from build123d import *

# Parameters (mm, degrees)
F1_DEPTH = 1.25
F3_DEPTH = 4.75
F5_DEPTH = 2


with BuildPart() as f1:
    # F0 (on Top) → F1 (new body)
    with BuildSketch(Plane.XY):
        with BuildLine():
            ThreePointArc((5.9976509575, 42.832122093), (6.6456632834, 42.7363739632), (7.2921511628, 42.6308225515))
            Line((7.2921511628, 42.6308225515), (7.5029069767, 43.8629272495))
            ThreePointArc((7.5029069767, 43.8629272495), (6.7010150496, 43.9925720697), (5.8968902794, 44.1075581395))
            ThreePointArc((5.8968902794, 44.1075581395), (5.9741669577, 43.5561736795), (6, 43))
            ThreePointArc((6, 43), (5.9994127106, 42.9160528296), (5.9976509575, 42.832122093))
        make_face()
        with BuildLine():
            Line((-7.5029069767, 43.8629272495), (-7.2921511628, 42.6308225515))
            ThreePointArc((-7.2921511628, 42.6308225515), (-6.6456632834, 42.7363739632), (-5.9976509575, 42.832122093))
            ThreePointArc((-5.9976509575, 42.832122093), (-5.9813637313, 43.4725335051), (-5.8968902794, 44.1075581395))
            ThreePointArc((-5.8968902794, 44.1075581395), (-6.7010150496, 43.9925720697), (-7.5029069767, 43.8629272495))
        make_face()
        with BuildLine():
            ThreePointArc((1.2281761729, 43.2325581395), (3.6184570865, 43.0983673509), (5.9976509575, 42.832122093))
            ThreePointArc((5.9976509575, 42.832122093), (5.9994127106, 42.9160528296), (6, 43))
            ThreePointArc((6, 43), (5.9741669577, 43.5561736795), (5.8968902794, 44.1075581395))
            ThreePointArc((5.8968902794, 44.1075581395), (0, 44.5), (-5.8968902794, 44.1075581395))
            ThreePointArc((-5.8968902794, 44.1075581395), (-5.9813637313, 43.4725335051), (-5.9976509575, 42.832122093))
            ThreePointArc((-5.9976509575, 42.832122093), (-3.6184570865, 43.0983673509), (-1.2281761729, 43.2325581395))
            ThreePointArc((-1.2281761729, 43.2325581395), (0, 44.25), (1.2281761729, 43.2325581395))
        make_face()
        with BuildLine():
            ThreePointArc((5.1487358592, 39.9193313953), (5.9687994799, 39.804973719), (6.7863372093, 39.6737712763))
            Line((6.7863372093, 39.6737712763), (7.2921511628, 42.6308225515))
            ThreePointArc((7.2921511628, 42.6308225515), (6.6456632834, 42.7363739632), (5.9976509575, 42.832122093))
            ThreePointArc((5.9976509575, 42.832122093), (5.7603447969, 41.3211826125), (5.1487358592, 39.9193313953))
        make_face()
        with BuildLine():
            ThreePointArc((-5.1487358592, 39.9193313953), (0, 40.25), (5.1487358592, 39.9193313953))
            ThreePointArc((5.1487358592, 39.9193313953), (5.7603447969, 41.3211826125), (5.9976509575, 42.832122093))
            ThreePointArc((5.9976509575, 42.832122093), (3.6184570865, 43.0983673509), (1.2281761729, 43.2325581395))
            ThreePointArc((1.2281761729, 43.2325581395), (1.244532084, 43.1167899479), (1.25, 43))
            ThreePointArc((1.25, 43), (-0.1167899479, 41.755467916), (-1.2281761729, 43.2325581395))
            ThreePointArc((-1.2281761729, 43.2325581395), (-3.6184570865, 43.0983673509), (-5.9976509575, 42.832122093))
            ThreePointArc((-5.9976509575, 42.832122093), (-5.7603447969, 41.3211826125), (-5.1487358592, 39.9193313953))
        make_face()
        with BuildLine():
            Line((-7.2921511628, 42.6308225515), (-6.7863372093, 39.6737712763))
            ThreePointArc((-6.7863372093, 39.6737712763), (-5.9687994799, 39.804973719), (-5.1487358592, 39.9193313953))
            ThreePointArc((-5.1487358592, 39.9193313953), (-5.7603447969, 41.3211826125), (-5.9976509575, 42.832122093))
            ThreePointArc((-5.9976509575, 42.832122093), (-6.6456632834, 42.7363739632), (-7.2921511628, 42.6308225515))
        make_face()
        with BuildLine():
            Line((-6.7863372093, 39.6737712763), (-6.5755813953, 38.4416665782))
            ThreePointArc((-6.5755813953, 38.4416665782), (-5.4165900946, 38.6220215906), (-4.2526993305, 38.7674418605))
            ThreePointArc((-4.2526993305, 38.7674418605), (-4.7358693269, 39.3160426552), (-5.1487358592, 39.9193313953))
            ThreePointArc((-5.1487358592, 39.9193313953), (-5.9687994799, 39.804973719), (-6.7863372093, 39.6737712763))
        make_face()
        with BuildLine():
            ThreePointArc((-4.2526993305, 38.7674418605), (0, 39), (4.2526993305, 38.7674418605))
            ThreePointArc((4.2526993305, 38.7674418605), (4.7358693269, 39.3160426552), (5.1487358592, 39.9193313953))
            ThreePointArc((5.1487358592, 39.9193313953), (0, 40.25), (-5.1487358592, 39.9193313953))
            ThreePointArc((-5.1487358592, 39.9193313953), (-4.7358693269, 39.3160426552), (-4.2526993305, 38.7674418605))
        make_face()
        with BuildLine():
            ThreePointArc((4.2526993305, 38.7674418605), (5.4165900946, 38.6220215906), (6.5755813953, 38.4416665782))
            Line((6.5755813953, 38.4416665782), (6.7863372093, 39.6737712763))
            ThreePointArc((6.7863372093, 39.6737712763), (5.9687994799, 39.804973719), (5.1487358592, 39.9193313953))
            ThreePointArc((5.1487358592, 39.9193313953), (4.7358693269, 39.3160426552), (4.2526993305, 38.7674418605))
        make_face()
        with BuildLine():
            ThreePointArc((6.7863372093, 39.6737712763), (7.3721720875, 39.5690987857), (7.9563953488, 39.4557761684))
            Line((7.9563953488, 39.4557761684), (8.5494186047, 42.3965793611))
            ThreePointArc((8.5494186046, 42.3965793611), (7.9216507524, 42.5183483846), (7.2921511628, 42.6308225515))
            Line((7.2921511628, 42.6308225515), (6.7863372093, 39.6737712763))
        make_face()
        with BuildLine():
            Line((-8.5494186047, 42.3965793611), (-7.9563953488, 39.4557761684))
            ThreePointArc((-7.9563953488, 39.4557761684), (-7.3721720874, 39.5690987857), (-6.7863372093, 39.6737712763))
            Line((-6.7863372093, 39.6737712763), (-7.2921511628, 42.6308225515))
            ThreePointArc((-7.2921511628, 42.6308225515), (-7.9216507524, 42.5183483846), (-8.5494186046, 42.3965793611))
        make_face()
    extrude(amount=F1_DEPTH)

    # F2 (on Top) → F3 (join)
    with BuildSketch(Plane.XY):
        with BuildLine():
            ThreePointArc((6.0348837209, 42.8268920011), (7.2953245865, 42.6302796047), (8.5494186046, 42.3965793611))
            Line((8.5494186047, 42.3965793611), (8.7965116279, 43.6219140247))
            ThreePointArc((8.7965116279, 43.6219140247), (7.5061721179, 43.8623686106), (6.2093023256, 44.0646634462))
            Line((6.2093023256, 44.0646634462), (6.0348837209, 42.8268920011))
        make_face()
        with BuildLine():
            Line((-8.7965116279, 43.6219140247), (-8.5494186047, 42.3965793611))
            ThreePointArc((-8.5494186046, 42.3965793611), (-7.2953245865, 42.6302796047), (-6.0348837209, 42.8268920011))
            Line((-6.0348837209, 42.8268920011), (-6.2093023256, 44.0646634462))
            ThreePointArc((-6.2093023256, 44.0646634462), (-7.5061721179, 43.8623686106), (-8.7965116279, 43.6219140247))
        make_face()
    extrude(amount=F3_DEPTH)

    # F4 (on Top) → F5 (join)
    with BuildSketch(Plane.XY):
        with BuildLine():
            Line((-7.9563953488, 39.4557761684), (-7.7093023256, 38.2304415048))
            ThreePointArc((-7.7093023256, 38.2304415048), (-7.1432226437, 38.3402447862), (-6.5755813953, 38.4416665782))
            Line((-6.5755813953, 38.4416665782), (-6.7863372093, 39.6737712763))
            ThreePointArc((-6.7863372093, 39.6737712763), (-7.3721720874, 39.5690987857), (-7.9563953488, 39.4557761684))
        make_face()
        with BuildLine():
            ThreePointArc((6.5755813953, 38.4416665782), (7.1432226437, 38.3402447862), (7.7093023256, 38.2304415048))
            Line((7.7093023256, 38.2304415048), (7.9563953488, 39.4557761684))
            ThreePointArc((7.9563953488, 39.4557761684), (7.3721720875, 39.5690987857), (6.7863372093, 39.6737712763))
            Line((6.7863372093, 39.6737712763), (6.5755813953, 38.4416665782))
        make_face()
    extrude(amount=F5_DEPTH)


solid = f1.part
Read the model definition and answer for the solid it produces. Units are mm, in the model's axes. A direction names the side the tool comes from. Give positions to 0.01 mm unless a question says otherwise; leave off trailing zeros. Write each loop counter-clockwise with the first axis right and the second up, starting at its lowest first coordinate (ties: lowest second). Pieces come first, ordered by that corner, then holes. Notation, with made-up numbers: (6.25, 87) - (14.25, 87) arc R17 ccw to (14.25, 109) - close; hole circle Ø11 at (75.5, 7). An arc over 180 degrees is marked (long way). Answer in a Markdown table with one row per item. Add a question column.
Item 1: Flat-ended cylindrical pins translate along their axes: P1, Ø3, axis at x = -2, y = 41, coming from the +Z side; P2, Ø1.5, axis at x = 7, y = 38.5, coming from the +Z side; P3, Ø2, axis at y = 39.5, z = 4, coming from the -X side; P4, Ø1.5, axis at x = -1, z = 1, coming from the -Y side. Find the tip coordinate at first contact, or state that the pin passes through.
Item 2: Section A-A, the plane x = 0 is taken. Write down the section's boundary in (y, z), and give its area (3 significant figures).
Item 3: Section C-C, the plane x = -4.5 is taken. Write down the section's boundary in (y, z).
Item 4: A tool of negligible diameter and unlimited length cuts with its end or side. For faces 1 (the face through (-0.1, 41.5, 1.25)), 2 (the face through (-7, 43, 4.75)), 3 (the face through (6.123, 43.454, 2.976)), 4 (the face through (-7, 39, 2)), 5 (the face through (0, 41, 0)), from which of +Z, -Z, +X, -X, +Y, -Y can it reach the whole face along a straight path? Write none if from no direction.
Item 5: Find the intervals of material crossed by L1, parallel to Y at x = 0, z = 0.35; L2, parallel to Z at x = 3, y = 42.5; L3, parallel to X at y = 43, z = 0.5, in increasing order.
Item 6: Section D-D, the plane x = -2.5 is taken. Write down the section's boundary in (y, z).
Item 7: Section B-B, the plane z = 2.95 is taken. Write down the section's boundary in (x, y), and give its area (3 significant figures).
Recorded:
| question | item | result |
|---|---|---|
| 1 | P1 | stops at z = 1.25 |
| 1 | P2 | stops at z = 2 |
| 1 | P3 | passes through |
| 1 | P4 | stops at y = 38.96 |
| 2 | outline | (39, 0) - (41.75, 0) - (41.75, 1.25) - (39, 1.25) - close; (44.25, 0) - (44.5, 0) - (44.5, 1.25) - (44.25, 1.25) - close |
| 2 | area | 3.75 mm2 |
| 3 | outline | (38.74, 0) - (44.27, 0) - (44.27, 1.25) - (38.74, 1.25) - close |
| 4 | face 1 | +Z |
| 4 | face 2 | +Z, +X, -X, +Y, -Y |
| 4 | face 3 | +Z, +Y |
| 4 | face 4 | +Z, +X, -X, -Y |
| 4 | face 5 | -Z, +X, -X, +Y, -Y |
| 5 | L1 | y = 39 to 41.75, 44.25 to 44.5 |
| 5 | L2 | z = 0 to 1.25 |
| 5 | L3 | x = -8.67 to -1.25, 1.25 to 8.67 |
| 6 | outline | (38.92, 0) - (44.43, 0) - (44.43, 1.25) - (38.92, 1.25) - close |
| 7 | outline | (-8.8, 43.62) - (-8.55, 42.4) arc R43.25 cw to (-6.03, 42.83) - (-6.21, 44.06) arc R44.5 ccw to start; (6.03, 42.83) arc R43.25 cw to (8.55, 42.4) - (8.8, 43.62) arc R44.5 ccw to (6.21, 44.06) - close |
| 7 | area | 6.47 mm2 |
